```python
from build123d import *

# Parameters (mm, degrees)
F1_DEPTH = 869.95
F3_DEPTH = 3.175
F5_DEPTH = 3.175
F7_D     = 9.525
F7_DEPTH = 5.08


with BuildPart() as f1:
    # F0 (on Front) → F1 (new body)
    with BuildSketch(Plane.XZ):
        Polygon((0, -38.1), (-50.8, 0), (-50.8, -3.96875), (0, -42.06875), (50.8, -3.96875), (50.8, 0), align=None)
        Polygon((-50.8, -3.96875), (-50.8, 0), (-53.975, 0), (-53.975, -42.06875), (-50.8, -42.06875), align=None)
    extrude(amount=-F1_DEPTH)

    # F2 (on face) → F3 (join)
    with BuildSketch(Plane(origin=(0, 869.95, 0), x_dir=(-1, 0, 0), z_dir=(0, 1, 0))):
        Polygon((50.8, 0), (-50.8, 0), (0, -38.1), align=None)
    extrude(amount=-F3_DEPTH)

    # F4 (on face) → F5 (join)
    with BuildSketch(Plane.XZ):
        Polygon((50.8, 0), (-50.8, 0), (0, -38.1), align=None)
    extrude(amount=-F5_DEPTH)

    # F7
    with Locations(Plane(origin=(-53.975, 0, 0), x_dir=(0, -1, 0), z_dir=(-1, 0, 0))):
        with Locations((-819.15, -21.034375), (-666.75, -21.034375), (-514.35, -21.034375), (-355.6, -21.034375), (-203.2, -21.034375), (-50.8, -21.034375)):
            Hole(F7_D / 2, depth=F7_DEPTH)


solid = f1.part
```
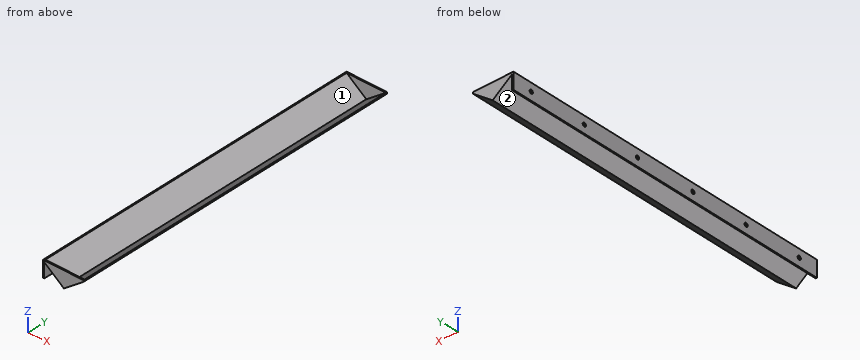
Input: part model. Units: mm. Frame: model coordinates. Face numbers are marked on the shaded views. Give positions to 0.01 mm unless a question says otherwise; leave off trailing zeros. Write each loop counter-clockwise with the first axis right and the second up, starting at its lowest first coordinate (ties: lowest second). Pieces come first, ordered by that corner, then holes. Notation, with made-up numbers: (17, -20.75) - (29, -20.75) arc R17 ccw to (29, -7.75) - close; hole circle Ø9 at (83.5, 5.5). An arc over 180 degrees is marked (long way). Write item = value, one per line. Start each with the question number.
1) Cut plane B-B (x = 10.5). Return loops of the section in (y, z) (3 decimals).
2) Pin query (flat end, axial travel): pin 1 (19 mm diameter, centred on y = 417, z = -18.5, fed in from +X); pin 2 (8.5 mm diameter, centred on y = 50.8, z = -21.03, fed in from +X); pin 3 (12 mm diameter, centred on x = -37.5, y = 604, fed in from +Z) (3 decimals). Return the tip coordinate at first contact, or that it passes through.
3) Draft query along Y for the marked faces 1 and 2. Return one class per face: pulls with the +Y half, pulls with the -Y half, needs draft (parallel to the pull), parting line crosses it, or undercut.
4) Cut plane A-A (y = 586). Return loops of the section in (x, z) (3 decimals), and give its area (3 significant figures).
5) Material intervals for L1, parallel to Y at x = 18.5, z = -10 (3 decimals); L2, parallel to Z at x = -52.3, y = 514.35; L3, parallel to X at y = 380, z = -14.5 (3 decimals), sorted ascending. Write a range as [from, to].
Answers follow:
q1.outline = (0, -34.194) - (869.95, -34.194) - (869.95, 0) - (866.775, 0) - (866.775, -30.225) - (3.175, -30.225) - (3.175, 0) - (0, 0) - close
q2.pin_1 = 44.09
q2.pin_2 = 33.72
q2.pin_3 = -5.475
q3.face_1 = undercut
q3.face_2 = needs draft
q4.outline = (-53.975, -42.069) - (-50.8, -42.069) - (-50.8, -3.969) - (0, -42.069) - (50.8, -3.969) - (50.8, 0) - (0, -38.1) - (-50.8, 0) - (-53.975, 0) - close
q4.area = 537 mm^2
q5.L1 = [0, 3.175], [866.775, 869.95]
q5.L2 = [-42.07, -25.8], [-16.27, 0]
q5.L3 = [-53.975, -50.8], [-36.758, -31.467], [31.467, 36.758]
